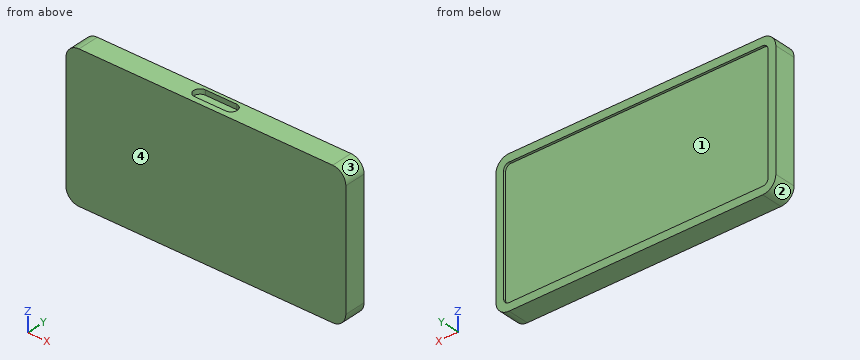
```python
from build123d import *

# Parameters (mm, degrees)
F0_W     = 151.638
F0_H     = 77.47
F1_DEPTH = 11.684
F2_R     = 7.112
F4_DEPTH = 2.667
F6_DEPTH = 1.27


with BuildPart() as f1:
    # F0 (on Front) → F1 (new body)
    with BuildSketch(Plane.XZ):
        with Locations((75.819, 38.735)):
            Rectangle(F0_W, F0_H)
    extrude(amount=F1_DEPTH)

    # F2
    f2_edges = [f1.edges().sort_by_distance(p)[0] for p in [
        (0, -5.842, 77.47),
        (151.638, -5.842, 77.47),
        (151.638, -5.842, 0),
        (0, -5.842, 0),
    ]]
    fillet(f2_edges, radius=F2_R)

    # F3 (on face) → F4 (cut)
    with BuildSketch(Plane.XY.offset(77.47)):
        with BuildLine():
            Line((83.947, -1.778), (67.183, -1.778))
            ThreePointArc((67.183, -1.778), (63.754, -5.207), (67.183, -8.636))
            Line((67.183, -8.636), (83.947, -8.636))
            ThreePointArc((83.947, -8.636), (87.376, -5.207), (83.947, -1.778))
        make_face()
    extrude(amount=-F4_DEPTH, mode=Mode.SUBTRACT)

    # F5 (on face) → F6 (cut)
    with BuildSketch(Plane(origin=(0, 0, 0), x_dir=(-1, 0, 0), z_dir=(0, 1, 0))):
        with BuildLine():
            Line((-147.447, 70.358), (-147.447, 7.112))
            ThreePointArc((-147.447, 7.112), (-146.591459, 5.046541), (-144.526, 4.191))
            Line((-144.526, 4.191), (-7.112, 4.191))
            ThreePointArc((-7.112, 4.191), (-5.046541, 5.046541), (-4.191, 7.112))
            Line((-4.191, 7.112), (-4.191, 70.358))
            ThreePointArc((-4.191, 70.358), (-5.046541, 72.423459), (-7.112, 73.279))
            Line((-7.112, 73.279), (-144.526, 73.279))
            ThreePointArc((-144.526, 73.279), (-146.591459, 72.423459), (-147.447, 70.358))
        make_face()
    extrude(amount=-F6_DEPTH, mode=Mode.SUBTRACT)


solid = f1.part
```
Verification items for the finished model (mm, model axes). Face numbers are marked on the shaded views. Give positions to 0.01 mm unless a question says otherwise; leave off trailing zeros. Order: outer loops, then holes, each group sorted by start corner. A loop starts at its lowest first (then second) coordinate and runs counter-clockwise, first axis right, second up. Notation, with made-up numbers: M -15.75,84.5 L 34.25,84.5 A13 ccw 34.25,109.5 Z; hole C 73.5,28.5 d4. An arc over 180 degrees is marked long. Return JSON: item names as keys, results as strings. Group by question number.
1) Scan lines: line 1 (Z direction, x = 88.5, y = -0.25); line 2 (Y direction, x = 145.5, z = 67); line 3 (X direction, y = -1, z = 17). Record each from-to range of solid material in increasing order.
2) Go/stop test with a flat-tipped pin: pin 1 Ø3.5 at (x, y) = (75.5, -6) entering from +Z. Record where the tip stops, or that it passes through.
3) Section check B-B on z = 19.5. Record the cut outline in (x, y), and give its area (3 significant figures).
4) Section check A-A on x = 91. Record the cut outline in (y, z).
5) Mould release check, pull along Z, two halves, no side actions. Record for the marked faces 1, 2, 3 and 4: pulls with the +Z half, pulls with the -Z half, needs draft (parallel to the pull), parting line crosses it, or undercut.
6) Section check C-C on x = 74. Record the cut outline in (y, z), and give its area (3 significant figures).
Answer block:
{
 "1": {"line 1": "z = 0 to 4.19, 73.28 to 77.47", "line 2": "y = -11.68 to -1.27", "line 3": "x = 0 to 4.19, 147.45 to 151.64"},
 "2": {"pin 1": "stops at z = 74.8"},
 "3": {"outline": "M 0,-11.68 L 151.64,-11.68 L 151.64,0 L 147.45,0 L 147.45,-1.27 L 4.19,-1.27 L 4.19,0 L 0,0 Z", "area": "1,590 mm^2"},
 "4": {"outline": "M -11.68,0 L 0,0 L 0,4.19 L -1.27,4.19 L -1.27,73.28 L 0,73.28 L 0,77.47 L -11.68,77.47 Z"},
 "5": {"face 1": "undercut", "face 2": "pulls with the -Z half", "face 3": "pulls with the +Z half", "face 4": "needs draft"},
 "6": {"outline": "M -11.68,0 L 0,0 L 0,4.19 L -1.27,4.19 L -1.27,73.28 L 0,73.28 L 0,77.47 L -1.78,77.47 L -1.78,74.8 L -8.64,74.8 L -8.64,77.47 L -11.68,77.47 Z", "area": "799 mm^2"}
}
